Could you check a few things on this model? Use its own coordinates, in mm. A direction names the side the tool comes from. Give positions to 0.01 mm unless a question says otherwise; leave off trailing zeros. Write each loop counter-clockwise with the first axis right and the second up, starting at its lowest first coordinate (ties: lowest second). Pieces come first, ordered by that corner, then holes. Notation, with made-up numbers: M 76,73 L 84,73 A22 cw 84,89 Z; hole C -5.5,84.5 d8. An arc over 180 degrees is marked long. Answer as a JSON object with one key per item and string values. Group by question number.
```python
from build123d import *

# Parameters (mm, degrees)
BOSS_EXTRUDE1_DEPTH      = 3.175
BOSS_EXTRUDE1_DEPTH_BACK = 3.175
CUT_EXTRUDE1_DEPTH       = 7.35
SKETCH3_R                = 1.5
CUT_EXTRUDE2_DEPTH       = 25
SKETCH4_R                = 1.75
CUT_EXTRUDE3_DEPTH       = 5
FILLET1_R                = 1


with BuildPart() as part:
    # Sketch1 → Boss-Extrude1 (new body, two sides)
    with BuildSketch(Plane.XY) as boss_extrude1_sk:
        with BuildLine():
            Line((136.313708499, 40.4), (122.825, 53.888708499))
            Line((122.825, 53.888708499), (122.825, 99))
            Line((122.825, 99), (124.470898034, 99))
            ThreePointArc((124.470898034, 99), (127.825, 101.5), (131.179101966, 99))
            Line((131.179101966, 99), (137.825, 99))
            Line((137.825, 99), (137.825, 40.4))
            Line((137.825, 40.4), (136.313708499, 40.4))
        make_face()
    extrude(amount=BOSS_EXTRUDE1_DEPTH)
    extrude(boss_extrude1_sk.sketch, amount=-BOSS_EXTRUDE1_DEPTH_BACK)

    # Sketch2 → Cut-Extrude1 (cut, through all)
    with BuildSketch(Plane.XY.offset(3.175)):
        with BuildLine():
            Line((125.725, 72), (125.725, 82))
            ThreePointArc((125.725, 82), (127.825, 84.1), (129.925, 82))
            Line((129.925, 82), (129.925, 72))
            ThreePointArc((129.925, 72), (127.825, 69.9), (125.725, 72))
        make_face()
        with BuildLine():
            Line((125.725, 88), (125.725, 98))
            ThreePointArc((125.725, 98), (127.825, 100.1), (129.925, 98))
            Line((129.925, 98), (129.925, 88))
            ThreePointArc((129.925, 88), (127.825, 85.9), (125.725, 88))
        make_face()
    extrude(amount=-CUT_EXTRUDE1_DEPTH, mode=Mode.SUBTRACT)

    # Sketch3 → Cut-Extrude2 (cut)
    with BuildSketch(Plane(origin=(0, 99, 0), x_dir=(1, 0, 0), z_dir=(0, 1, 0))):
        with Locations((133.825, 0)):
            Circle(SKETCH3_R)
    extrude(amount=-CUT_EXTRUDE2_DEPTH, mode=Mode.SUBTRACT)

    # Sketch4 → Cut-Extrude3 (cut)
    with BuildSketch(Plane(origin=(0, 99, 0), x_dir=(-1, 0, 0), z_dir=(0, 1, 0))):
        with Locations((-133.825, 0)):
            Circle(SKETCH4_R)
    extrude(amount=-CUT_EXTRUDE3_DEPTH, mode=Mode.SUBTRACT)

    # Fillet1
    fillet1_edges = [part.edges().sort_by_distance(p)[0] for p in [
        (124.470898034, 99, 0),
        (131.179101966, 99, 0),
    ]]
    fillet(fillet1_edges, radius=FILLET1_R)


solid = part.part
```
1) If we section it at B-B, the plane z = 0: List the corners of the cut face in (x, y) for me (3 decimals), plus the area to 3 significant figures.
2) If we section it at A-A, the plane y = 75.5: List the corners of the cut face in (x, z) for me (3 decimals).
3) If we section it at D-D, the plane x = 134.5: List the corners of the cut face in (y, z) for me (3 decimals), plus the area to 3 significant figures.
4) For faces 4 (the flat face through (130, 71, 3.175)), 5 (the flat face through (123, 99, 0)), 6 (the cylindrical face through (132.156, 96.535, 0.526)), 7 (the cylindrical face through (127.8, 100.1, 0)), which set-ups out of +Z, -Z, +X, -X, +Y, -Y let a thin tool reach every point of the face, with its end or its side?
5) If we section it at C-C, the plane x = 127: List the corners of the cut face in (y, z) for me (3 decimals).
6) Please list where these lines run through material, in increasing order: line 1 along X through (y, z) = (80.5, 0) (3 decimals); line 2 along Y through (x, z) = (129.5, 1); line 3 along Y through (x, z) = (128, 1.5). Write a range as from..to.
7) We'd pull the mould along Y, two halves only. Please class faces 1 (the flat face through (136, 99, 0)), 2 (the flat face through (129.925, 77, 0)), 3 (the flat face through (137, 40.4, 0)): released by +Y, released by -Y, zero draft, split by the parting line, or undercut.
8) I'm going to push flat-ended pins straight in: pin 1 (3.5 mm diameter, centred on x = 134.5, z = 0, fed in from +Y); pin 2 (1 mm diameter, centred on x = 134, z = -0.5, fed in from +Y); pin 3 (3.5 mm diameter, centred on x = 133.825, z = 0, fed in from -Y). Where does each tip first touch, or does it pass through?
Taken from the geometry:
{
 "1": {"outline": "M 122.825,53.889 L 136.314,40.4 L 137.825,40.4 L 137.825,99 L 135.575,99 L 135.575,94 L 135.325,94 L 135.325,74 L 132.325,74 L 132.325,94 L 132.075,94 L 132.075,99 L 131.856,99 A1 cw 130.96,99.556 A3.5 ccw 124.69,99.556 A1 cw 123.794,99 L 122.825,99 Z; hole M 125.725,72 A2.1 ccw 129.925,72 L 129.925,82 A2.1 ccw 125.725,82 Z; hole M 125.725,88 A2.1 ccw 129.925,88 L 129.925,98 A2.1 ccw 125.725,98 Z", "area": "611 mm²"},
 "2": {"outline": "M 122.825,-3.175 L 125.725,-3.175 L 125.725,3.175 L 122.825,3.175 Z; M 129.925,-3.175 L 137.825,-3.175 L 137.825,3.175 L 129.925,3.175 Z; hole C 133.825,0 d3"},
 "3": {"outline": "M 42.214,-3.175 L 99,-3.175 L 99,-1.615 L 94,-1.615 L 94,-1.34 L 74,-1.34 L 74,1.34 L 94,1.34 L 94,1.615 L 99,1.615 L 99,3.175 L 42.214,3.175 Z", "area": "291 mm²"},
 "4": {"face 4": "+Z, +X, -X, +Y, -Y", "face 5": "+Z, -Z, -X, +Y", "face 6": "+Y", "face 7": "+Z, -Z"},
 "5": {"outline": "M 49.714,-3.175 L 70.069,-3.175 L 70.069,3.175 L 49.714,3.175 Z; M 83.931,-3.175 L 86.069,-3.175 L 86.069,3.175 L 83.931,3.175 Z; M 99.931,-3.175 L 101.401,-3.175 L 101.401,3.175 L 99.931,3.175 Z"},
 "6": {"line 1": "122.825..125.725, 129.925..132.325, 135.325..137.825", "line 2": "47.21..70.73, 83.27..86.73, 99.27..101.07", "line 3": "48.71..69.91, 84.09..85.91, 100.09..101.5"},
 "7": {"face 1": "released by +Y", "face 2": "undercut", "face 3": "released by -Y"},
 "8": {"pin 1": "y = 99", "pin 2": "y = 74", "pin 3": "y = 41.14"}
}
